```python
from build123d import *

# Parameters (mm, degrees)
SKETCH2_R          = 3.1242
CUT_EXTRUDE1_DEPTH = 20.05


with BuildPart() as part:
    # Sketch1 → Revolve1 (revolve)
    with BuildSketch(Plane.XY):
        Polygon((0, 0), (19.05, 0), (19.05, 31.75), (16.51, 31.75), (16.51, 19.05), (7.62, 19.05), (7.62, 31.75), (5.08, 31.75), (5.08, 6.35), (0, 6.35), align=None)
    revolve(axis=Axis((0, 0, 0), (1, 0, 0)))

    # Sketch2 → Cut-Extrude1 (cut, through all)
    with BuildSketch(Plane.ZY):
        Circle(SKETCH2_R)
    extrude(amount=-CUT_EXTRUDE1_DEPTH, mode=Mode.SUBTRACT)


solid = part.part
```
Can you work these out from the model? Positions are in its coordinate system, mm. A direction names the side the tool comes from. Round coordinates to 2 decimals unless told otherwise and drop trailing zeros. Loops run counter-clockwise (first coordinate to the right, second up) from the corner with the lowest first, then second, coordinate; pieces in that order, holes last. Notation, with made-up numbers: (77.5, 63) -> (119.5, 63) arc R10 cw to (119.5, 68) -> close; hole circle Ø5 at (25.5, 40.25). An arc over 180 degrees is marked (long way). One line per item, written item: value. Start each with the question number.
1. For faces 1 (the cylindrical face through (2.5, -1.38, -6.2)), 2 (the cylindrical face through (17.762, -6.883, -30.995)), 3 (the cylindrical face through (12, -15.12, -11.59)), which set-ups out of +Z, -Z, +X, -X, +Y, -Y let a thin tool reach every point of the face, with its end or its side?
2. If we mould it in two halves opening along X, with no side actions, what happens to faces 4 (the flat face through (19.05, -7, 0)), 5 (the flat face through (7.62, -14, -14)), 6 (the cylindrical face through (6.332, -6.883, -30.995)), 7 (the flat face through (16.51, 14, -14))? For each: pulls with the +X half, pulls with the -X half, needs draft (parallel to the pull), parting line crosses it, or undercut.
3. If we section it at C-C, the plane x = 18: Write out the boundary of the cut face in (y, z).
4. For pin 1 (3 mm diameter, centred on x = 2, z = 25, fed in from +Y); pin 2 (3 mm diameter, centred on x = 11.5, z = -10.5, fed in from -Y); pin 3 (1 mm diameter, centred on x = 12.5, y = -3, fed in from -Z); pin 4 (8 mm diameter, centred on y = 10, z = 9, fed in from -X), each with a flat end and sliding along its axis, tell me the tip position at first contact or that it passes through.
5. If I drill on probe 1 along X at (y, z) = (12, 23); probe 2 along X at (y, z) = (9, -8.5); probe 3 along Z at (x, y) = (9.5, 2), over which ranges is the centre line in solid material (lowest first)?
6. If we section it at A-A, the plane z = 0: Write out the boundary of the cut face in (x, y).
7. If we section it at D-D, the plane y = 8: Write out the boundary of the cut face in (x, z), then the cut area to 3 significant figures.
Calculated:
1. face 1: -X
1. face 2: +X, -X
1. face 3: none
2. face 4: pulls with the +X half
2. face 5: undercut
2. face 6: needs draft
2. face 7: undercut
3. outline: circle Ø63.5 at (0, 0); hole circle Ø6.25 at (0, 0)
4. pin 1: passes through
4. pin 2: stops at y = -16.79
4. pin 3: stops at z = -18.89
4. pin 4: stops at x = 5.08
5. probe 1: x = 5.08 to 7.62, 16.51 to 19.05
5. probe 2: x = 5.08 to 19.05
5. probe 3: z = -18.94 to -2.4, 2.4 to 18.94
6. outline: (0, -6.35) -> (5.08, -6.35) -> (5.08, -31.75) -> (7.62, -31.75) -> (7.62, -19.05) -> (16.51, -19.05) -> (16.51, -31.75) -> (19.05, -31.75) -> (19.05, -3.12) -> (0, -3.12) -> close; (0, 3.12) -> (19.05, 3.12) -> (19.05, 31.75) -> (16.51, 31.75) -> (16.51, 19.05) -> (7.62, 19.05) -> (7.62, 31.75) -> (5.08, 31.75) -> (5.08, 6.35) -> (0, 6.35) -> close
7. outline: (5.08, -30.73) -> (7.62, -30.73) -> (7.62, -17.29) -> (16.51, -17.29) -> (16.51, -30.73) -> (19.05, -30.73) -> (19.05, 30.73) -> (16.51, 30.73) -> (16.51, 17.29) -> (7.62, 17.29) -> (7.62, 30.73) -> (5.08, 30.73) -> close
7. area: 620 mm²
